The listing builds one solid part. Answer for the finished solid, in the listing's coordinates (mm). Face numbers are marked on the shaded views. A direction names the side the tool comes from. Round coordinates to 2 decimals unless told otherwise and drop trailing zeros. Order: outer loops, then holes, each group sorted by start corner. A loop starts at its lowest first (then second) coordinate and runs counter-clockwise, first axis right, second up. Notation, with made-up numbers: M 65.25,-34 L 107.25,-34 A25 ccw 107.25,-6 Z; hole C 39,55 d10. An arc over 180 degrees is marked long. Write item = value, one per line. Start each with the question number.
(1) For a pull along Z with two mould halves and no side action, classify the marked faces 1, 2 and 3 as released by +Z, released by -Z, zero draft, split by the parting line, or undercut.
(2) A cutting plane is placed at B-B, the plane x = 5.5. Determine the outline of the cut face in (y, z).
(3) Straight lines are drawn through the part: probe 1 along X at (y, z) = (1.15, -1); probe 2 along Z at (x, y) = (-17.5, 1.9); probe 3 along X at (y, z) = (6.75, 5). For each, find the intervals that lie inside material, in ascending order. Write a range as from..to.
(4) Each of these flat-tipped pins is pushed along its axis until it touches: pin 1 (0.9 mm diameter, centred on x = -34, z = -9, fed in from +Y); pin 2 (2.5 mm diameter, centred on x = 18.5, y = 2, fed in from -Z); pin 3 (2.5 mm diameter, centred on x = 28.5, y = 3, fed in from +Z); pin 4 (3 mm diameter, centred on x = -17.5, z = -1, fed in from +Y). Where does it stop, or does it pass through?
(5) A cutting plane is placed at C-C, the plane z = 3. Determine the outline of the cut face in (x, y), and give its area (3 significant figures).
(6) A cutting plane is placed at D-D, the plane x = 33. Determine the outline of the cut face in (y, z).
(7) Which of the six approach directions +Z, -Z, +X, -X, +Y, -Y give full straight-line access (tool end or side, diameter ignored) to the marked faces 4, 5, 6 and 7?
(8) A cutting plane is placed at A-A, the plane z = -10. Determine the outline of the cut face in (x, y).
from build123d import *

# Parameters (mm, degrees)
SKETCH1_W            = 31
SKETCH1_H            = 38
SKETCH1_W_2          = 29
SKETCH1_H_2          = 32
BOSS_EXTRUDE1_DEPTH  = 10
SKETCH2_W            = 6
SKETCH2_H            = 10
SKETCH2_R            = 2
BOSS_EXTRUDE2_DEPTH  = 3
SKETCH3_W            = 6
SKETCH3_H            = 3
CUT_EXTRUDE1_DEPTH   = 5
SKETCH4_W            = 29.5
SKETCH4_H            = 3
BOSS_EXTRUDE3_DEPTH  = 5
FILLET1_R            = 1
CHAMFER1_SIZE        = 8
FILLET1_OF_MIRROR2_R = 1


with BuildPart() as part:
    # Sketch1 → Boss-Extrude1 (new body)
    with BuildSketch(Plane(origin=(0, 0, 0), x_dir=(1, 0, 0), z_dir=(0, 1, 0))):
        Rectangle(SKETCH1_W, SKETCH1_H)
        Rectangle(SKETCH1_W_2, SKETCH1_H_2, mode=Mode.SUBTRACT)
    extrude(amount=BOSS_EXTRUDE1_DEPTH)

    # Sketch2 → Boss-Extrude2 (add)
    with BuildSketch(Plane.XZ):
        with Locations((17.5, -1)):
            Rectangle(SKETCH2_W, SKETCH2_H)
        with Locations(Location((17.5, -1, 0), (0, 0, 270))):
            Circle(SKETCH2_R, mode=Mode.SUBTRACT)
    boss_extrude2 = extrude(amount=-BOSS_EXTRUDE2_DEPTH)

    # Mirror1: Boss-Extrude2 across plane
    add(boss_extrude2.mirror(Plane(origin=(0, 0, 0), x_dir=(0, 0, 1), z_dir=(1, 0, 0))))

    # Sketch3 → Cut-Extrude1 (cut)
    with BuildSketch(Plane.XZ):
        with Locations((0, 17.5)):
            Rectangle(SKETCH3_W, SKETCH3_H)
    extrude(amount=-CUT_EXTRUDE1_DEPTH, mode=Mode.SUBTRACT)

    # Sketch4 → Boss-Extrude3 (add)
    with BuildSketch(Plane.XZ):
        Polygon((13.981367518, 33.29919815), (16.800445381, 32.27313772), (11.969418335, 19), (8.776885018, 19), align=None)
        with Locations((30.25, -9.5)):
            Rectangle(SKETCH4_W, SKETCH4_H)
    boss_extrude3 = extrude(amount=-BOSS_EXTRUDE3_DEPTH)

    # Fillet1
    fillet1_edges = [part.edges().sort_by_distance(p)[0] for p in [
        (10.373151677, 5, 19),
        (11.969418335, 2.5, 19),
    ]]
    fillet(fillet1_edges, radius=FILLET1_R)

    # Chamfer1
    chamfer1_edges = [part.edges().sort_by_distance(p)[0] for p in [
        (15.5, 5, -19),
        (-15.5, 5, -19),
        (14.5, 5, -16),
        (-14.5, 5, -16),
    ]]
    chamfer(chamfer1_edges, length=CHAMFER1_SIZE)

    # Mirror2: Boss-Extrude3 across plane
    add(boss_extrude3.mirror(Plane(origin=(0, 0, 0), x_dir=(0, 0, 1), z_dir=(1, 0, 0))))

    # Fillet1 of Mirror2
    fillet1_of_mirror2_edges = [part.edges().sort_by_distance(p)[0] for p in [
        (-10.373151677, 5, 19),
        (-11.969418335, 2.5, 19),
    ]]
    fillet(fillet1_of_mirror2_edges, radius=FILLET1_OF_MIRROR2_R)


solid = part.part
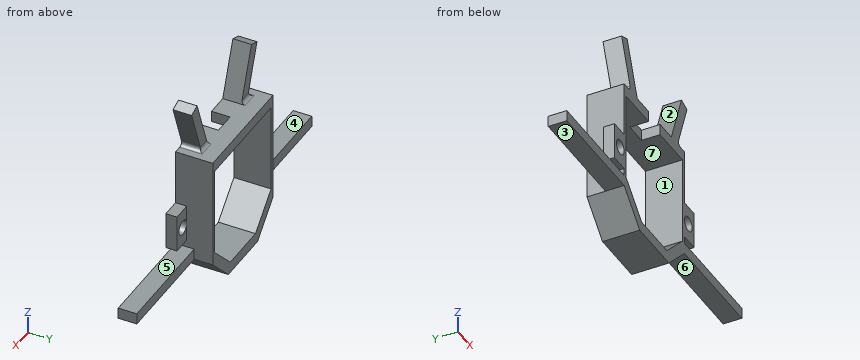
Reported:
q1.face_1 = undercut
q1.face_2 = released by +Z
q1.face_3 = released by -Z
q2.outline = M 0,-19 L 10,-19 L 10,-16 L 0,-16 Z; M 0,16 L 10,16 L 10,19 L 0,19 Z
q3.probe_1 = -20.5..-19.5, -15.5..-14.5, 14.5..15.5, 19.5..20.5
q3.probe_2 = -11..-8, -6..-3, 1..4
q3.probe_3 = -15.5..-14.5, 14.5..15.5
q4.pin_1 = 5
q4.pin_2 = -11
q4.pin_3 = -8
q4.pin_4 = through
q5.outline = M -20.5,0 L -14.5,0 L -14.5,10 L -15.5,10 L -15.5,3 L -20.5,3 Z; M 14.5,0 L 20.5,0 L 20.5,3 L 15.5,3 L 15.5,10 L 14.5,10 Z
q5.area = 50.0 mm²
q6.outline = M 0,-11 L 5,-11 L 5,-8 L 0,-8 Z
q7.face_4 = -X, +Y, -Y
q7.face_5 = +X, +Y, -Y
q7.face_6 = -Z, +X, +Y, -Y
q7.face_7 = +Y, -Y
q8.outline = M -45,0 L -12.5,0 L -12.5,10 L -15.5,10 L -15.5,5 L -45,5 Z; M 12.5,0 L 45,0 L 45,5 L 15.5,5 L 15.5,10 L 12.5,10 Z
